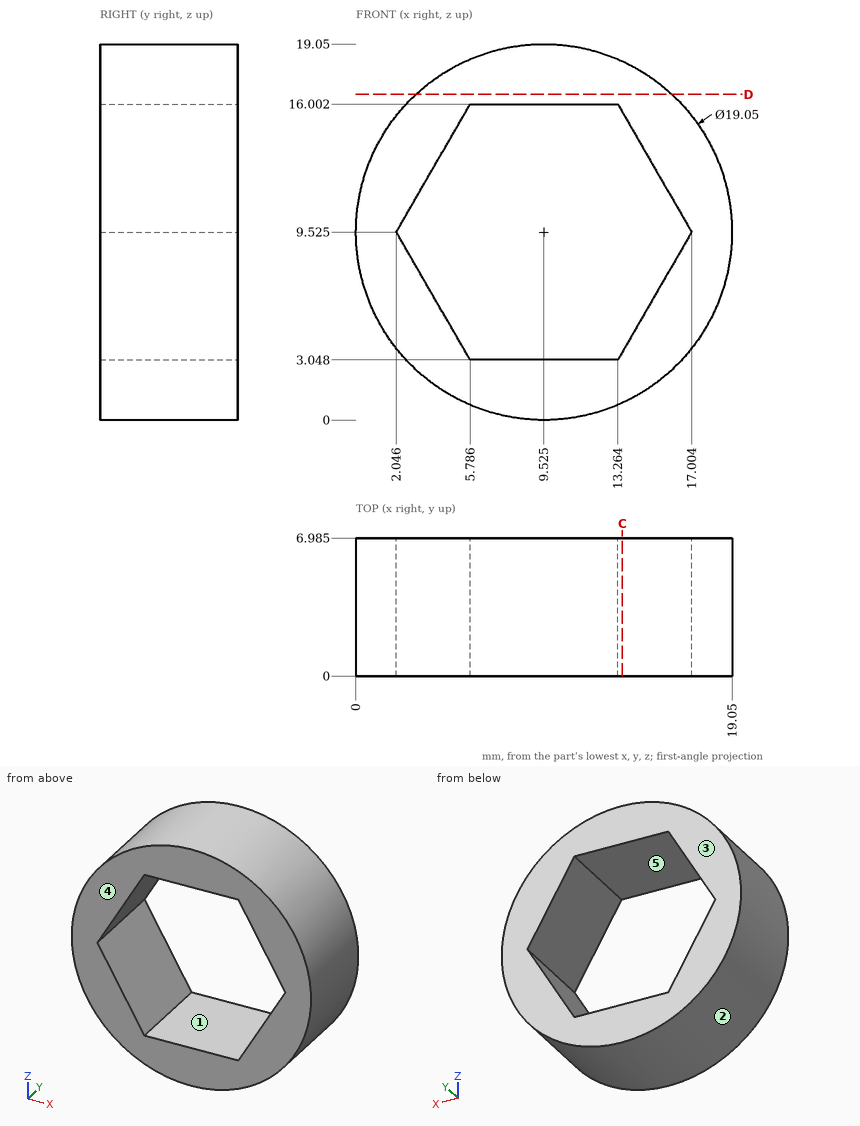
Design review of the part shown in the three views and the two pictorial views. Dimensions are in mm from the part's minimum x, y and z. A direction names the side the tool comes from. Coordinates: 2 decimals unless noted, no trailing zeros. Order: outer loops, then holes, each group sorted by start corner. A loop starts at its lowest first (then second) coordinate and runs counter-clockwise, first axis right, second up.
Item 1: Take a section at C-C, the plane x = 13.5. Write out the cut boundary in (y, z) (1 decimal).
Item 2: Take a section at D-D, the plane z = 16.5. Write out the cut boundary in (x, y) (1 decimal).
Item 3: For the marked faces 4 and 5, list the 3-axis set-ups (+Z, -Z, +X, -X, +Y, -Y) from which the entire face can be reached by the end or side of a thin tool; tool diameter is ignored.
Item 4: For line 1 (Z direction, x = 9.25, y = 6.5) (1 decimal); line 2 (Z direction, x = 14.25, y = 0.5) (1 decimal); line 3 (X direction, y = 4.5, z = 5.5), list the stretches that pass through material, from the lowest coordinate up.
Item 5: For pin 1 Ø1.5 at (y, z) = (2.5, 16) entering from -X; pin 2 Ø1 at (x, y) = (4.5, 1.5) entering from +Z; pin 3 Ø4 at (x, y) = (3, 0.5) entering from -Z, all flat-tipped, find the tip position at first contact; note any pin that passes through.
Item 6: The part is to be moulded in two halves that separate along X. For the marked faces 1, 2 and 3, say which applies: pulls with the +X half, pulls with the -X half, needs draft (parallel to the pull), parting line crosses it, or undercut.
The answers:
1. outline: (0, 0.9) - (7, 0.9) - (7, 3.5) - (0, 3.5) - close; (0, 15.6) - (7, 15.6) - (7, 18.2) - (0, 18.2) - close
2. outline: (3, 0) - (16, 0) - (16, 7) - (3, 7) - close
3. face 4: +Z, -Z, +X, -X, -Y
3. face 5: +Y, -Y
4. line 1: z = 0 to 3, 16 to 19
4. line 2: z = 1.3 to 4.8, 14.3 to 17.8
4. line 3: x = 0.89 to 4.37, 14.68 to 18.16
5. pin 1: stops at x = 1.91
5. pin 2: stops at z = 17.91
5. pin 3: stops at z = 1.14
6. face 1: undercut
6. face 2: parting line crosses it
6. face 3: needs draft
